Source: CAD feature listing. Evaluate the final solid. Frame: model axes, mm. Face numbers are marked on the shaded views. Give positions to 0.01 mm unless a question says otherwise; leave off trailing zeros. Loops run counter-clockwise (first coordinate to the right, second up) from the corner with the lowest first, then second, coordinate; pieces in that order, holes last. Notation, with made-up numbers: (-30.5, 3.25) -> (-21.5, 3.25) arc R17 cw to (-21.5, 18.25) -> close; hole circle Ø2 at (5.5, 51.25). An arc over 180 degrees is marked (long way). Put each result on its own line as item: value.
```python
from build123d import *

# Parameters (mm, degrees)
PAD001_DEPTH        = 30
SKETCH002_W         = 10
SKETCH002_H         = 65
PAD002_DEPTH        = 2
PAD003_DEPTH        = 2.25
BODY001_PITCH_ANGLE = 4.34


with BuildPart() as part:
    # Sketch001 (on DatumPlane) → Pad001 (new body)
    with BuildSketch(Plane.YZ.offset(31)):
        Polygon((-1, 2), (1, 2), (1, 1.25), (2.25, 0), (-2.25, 0), (-1, 1.25), align=None)
    extrude(amount=PAD001_DEPTH)

    # Sketch002 (on DatumPlane) → Pad002 (join)
    with BuildSketch(Plane(origin=(31, 0, 2), x_dir=(0, -1, 0), z_dir=(0, 0, 1))):
        with Locations((0, -0.65176)):
            Rectangle(SKETCH002_W, SKETCH002_H)
    extrude(amount=PAD002_DEPTH)

    # Sketch003 (on DatumPlane) → Pad003 (join, symmetric)
    with BuildSketch(Plane.XZ):
        Polygon((1, 2), (1, 0), (2, 0), (5.464102, 2), align=None)
    extrude(amount=PAD003_DEPTH, both=True)


with BuildPart() as part_1:
    # Body001 pitch: moved
    add(part.part.rotate(Axis((0, 0, 0), (0, 1, 0)), BODY001_PITCH_ANGLE))


with BuildPart() as part_2:
    # Body001 placement: moved
    add(part_1.part.moved(Location((3, 0, 43))))


solid = part_2.part
```
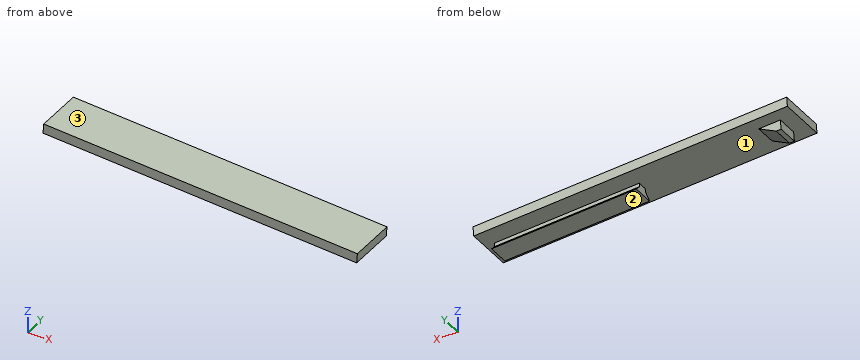
(1) Draft query along X for the marked faces 1, 2 and 3. Return one class per face: released by +X, released by -X, zero draft, split by the parting line, or undercut.
Calculated:
face 1: undercut
face 2: released by -X
face 3: released by +X
(2) Section D-D on x = 51. Return loops of the section in (y, z), then the cut area to 3 significant figures.
Calculated:
outline: (-5, 41.36) -> (-1, 41.36) -> (-1, 40.61) -> (-2.25, 39.36) -> (2.25, 39.36) -> (1, 40.61) -> (1, 41.36) -> (5, 41.36) -> (5, 43.37) -> (-5, 43.37) -> close
area: 25.6 mm²
(3) Section A-A on y = -0.25. Return loops of the section in (x, z), then the cut area to 3 significant figures.
Calculated:
outline: (1.01, 45.16) -> (4.15, 44.92) -> (4, 42.92) -> (4.99, 42.85) -> (8.6, 44.58) -> (34.06, 42.65) -> (33.91, 40.65) -> (63.83, 38.38) -> (63.98, 40.38) -> (65.82, 40.24) -> (65.97, 42.23) -> (1.16, 47.15) -> close
area: 195 mm²
(4) Section B-B on x = 6.5. Return loops of the section in (y, z), then the cut area to 3 significant figures.
Calculated:
outline: (-5, 44.74) -> (-2.25, 44.74) -> (-2.25, 43.57) -> (2.25, 43.57) -> (2.25, 44.74) -> (5, 44.74) -> (5, 46.75) -> (-5, 46.75) -> close
area: 25.3 mm²
(5) First-contact query: P1, Ø4, axis at x = 57.5, y = 3.5, coming from the -Z side; P2, Ø2, axis at x = 22, z = 41, coming from the -Y side; P3, Ø2, axis at y = -2.5, z = 43.5, coming from the -X side; P4, Ø1.7, axis at x = 7, z = 43.5, coming from the -Y side. Flat tips, straight axial feed; report the tip coordinate or a pass-through.
Calculated:
P1: stops at z = 38.75
P2: passes through
P3: stops at x = 4
P4: stops at y = -2.25
(6) Section C-C on z = 46. Return loops of the section in (x, y).
Calculated:
outline: (1.07, -5) -> (16.33, -5) -> (16.33, 5) -> (1.07, 5) -> close
(7) Line query: probe 1 along Z at (x, y) = (63, -1.5); probe 2 along Z at (x, y) = (55, 3.5); probe 3 along Z at (x, y) = (24.5, 0). Output: solid intervals per line, ascending. Write a range as from..to.
Calculated:
probe 1: z = 38.45..39.2, 40.45..42.46
probe 2: z = 41.06..43.07
probe 3: z = 43.37..45.38
